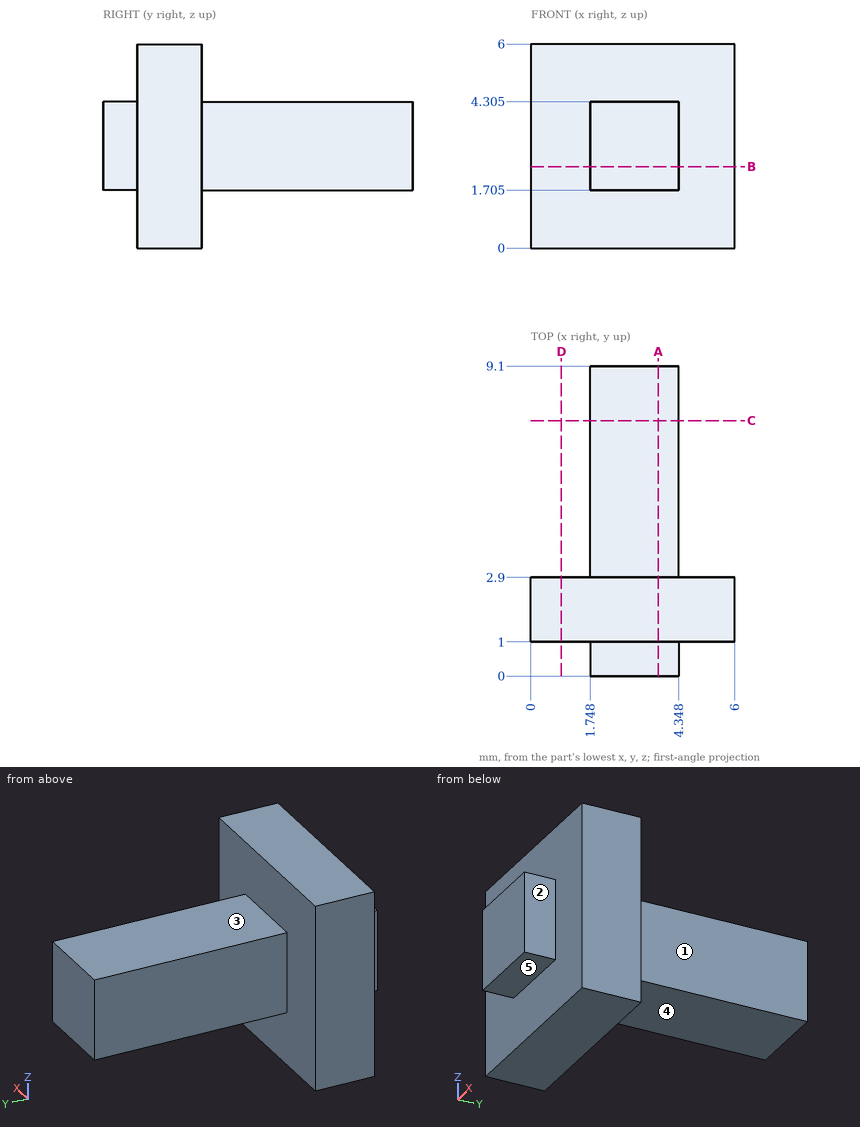
Geometry check sheet. Reference: drawing and pictorial views, mm from the part's lowest x, y, z. A direction names the side the tool comes from. Coordinates: 2 decimals unless noted, no trailing zeros. Write each loop counter-clockwise with the first axis right and the second up, starting at its lowest first coordinate (ties: lowest second). Pieces come first, ordered by that corner, then holes. Notation, with made-up numbers: (28, 26.25) - (84, 26.25) arc R12 cw to (84, 31.25) - close; hole circle Ø8 at (51, 79). An arc over 180 degrees is marked (long way). One line per question, with ' | ' between items. Start each with the question number.
1. Section check C-C (y = 7.5). Enter the section's corners in (x, z) (1 decimal).
2. Section check D-D (x = 0.9). Enter the section's corners in (y, z).
3. Access from +Z, -Z, +X, -X, +Y, -Y to the whole of each face (thin tool, end or side, straight path). Record for the marked faces 1, 2, 3, 4 and 5.
4. Section check B-B (z = 2.4). Enter the section's corners in (x, y).
5. Material ranges on line 1 along Z through (x, y) = (2.65, 6) (1 decimal); line 2 along X through (y, z) = (8, 3.7); line 3 along Y through (x, z) = (3.65, 0.35), recorded low to high.
6. Section check A-A (x = 3.75). Enter the section's corners in (y, z) (1 decimal).
7. Gauge pin test, flat ends, axial feed: P1, Ø1.3, axis at x = 3.5, y = 6.5, coming from the +Z side (1 decimal); P2, Ø2, axis at y = 1, z = 1.5, coming from the -X side; P3, Ø0.8, axis at y = 7, z = 3, coming from the -X side; P4, Ø2, axis at x = 2.5, y = 6.5, coming from the -Z side (1 decimal). Record the tip position at first contact, or that the pin passes through.
Computed values:
1) outline: (1.7, 1.7) - (4.3, 1.7) - (4.3, 4.3) - (1.7, 4.3) - close
2) outline: (1, 0) - (2.9, 0) - (2.9, 6) - (1, 6) - close
3) face 1: +Z, -Z, +X, +Y | face 2: +Z, -Z, +X, -Y | face 3: +Z, +X, -X, +Y | face 4: -Z, +X, -X, +Y | face 5: -Z, +X, -X, -Y
4) outline: (0, 1) - (1.75, 1) - (1.75, 0) - (4.35, 0) - (4.35, 1) - (6, 1) - (6, 2.9) - (4.35, 2.9) - (4.35, 9.1) - (1.75, 9.1) - (1.75, 2.9) - (0, 2.9) - close
5) line 1: 1.7 to 4.3 | line 2: 1.75 to 4.35 | line 3: 1 to 2.9
6) outline: (0, 1.7) - (1, 1.7) - (1, 0) - (2.9, 0) - (2.9, 1.7) - (9.1, 1.7) - (9.1, 4.3) - (2.9, 4.3) - (2.9, 6) - (1, 6) - (1, 4.3) - (0, 4.3) - close
7) P1: z = 4.3 | P2: x = 0 | P3: x = 1.75 | P4: z = 1.7
